Check sheet for the modelled part. Datum: model origin and axes. Units: mm. Face numbers are marked on the shaded views. Give positions to 0.01 mm unless a question says otherwise; leave off trailing zeros. Loops run counter-clockwise (first coordinate to the right, second up) from the corner with the lowest first, then second, coordinate; pieces in that order, holes last. Notation, with made-up numbers: (35, -5.75) - (73, -5.75) arc R34 ccw to (73, 27.25) - close; hole circle Ø7 at (-20, -3.75). An arc over 180 degrees is marked (long way). Use one line per item in the form item = value.
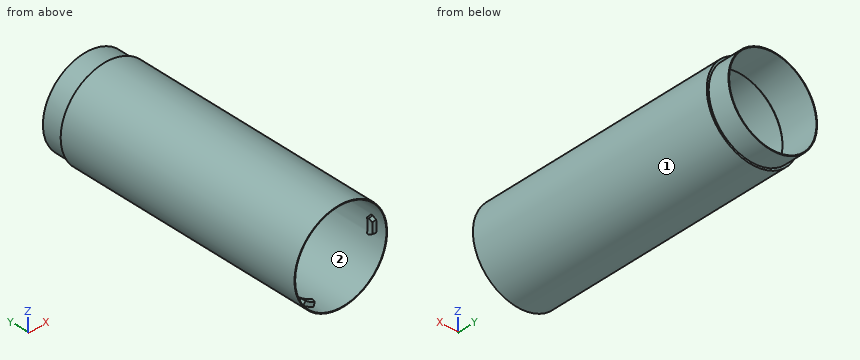
Autodesk Inventor part; units mm, degrees
ref_plane "Work Plane2" through (35, 0, 0) normal (1, 0, 0) x (0, 1, 0)
ref_plane "Work Plane4" through (34, 0, 0) normal (1, 0, 0) x (0, 1, 0)
ref_plane "Work Plane5" through (0, 8, 0) normal (0, -1, 0) x (1, 0, 0)
sketch "Sketch1" plane through (0, 0, 0) normal (0, 1, 0) x (-1, 0, 0)
  circle A0 centre (0, 0) radius 35
  circle A1 centre (0, 0) radius 34.5
  dimension "d0" = 70
  dimension "d1" = 69
extrude "Extrusion1" add sketch "Sketch1" along normal blind 189.5
ref_plane "Work Plane2" through (35, 0, 0) normal (1, 0, 0) x (0, 1, 0)
sketch "Sketch5" plane through (0, 189.5, 0) normal (0, 1, 0) x (1, 0, 0)
  circle A0 centre (0, 0) radius 33.5
  circle A1 centre (0, 0) radius 33
  dimension "d44" = 67
  dimension "d45" = 66
extrude "Extrusion3" add sketch "Sketch5" along normal blind 16
sketch "Sketch6" plane through (0, 189.5, 0) normal (0, -1, 0) x (1, 0, 0)
  circle A0 centre (0, 0) radius 33
  circle A1 centre (0, 0) radius 34.5
  circle A2 centre (0, 0) radius 34.5
  dimension "d112" = 66
  dimension "d113" = 69
extrude "Extrusion4" add sketch "Sketch6" along normal blind 12.5
ref_plane "Work Plane4" through (34, 0, 0) normal (1, 0, 0) x (0, 1, 0)
ref_plane "Work Plane5" through (0, 8, 0) normal (0, -1, 0) x (1, 0, 0)
sketch "Sketch11" plane through (0, 8, 0) normal (0, -1, 0) x (1, 0, 0)
  line L0 (0, 0) -> (37.8059, -6.6662) construction
  line L1 (37.8059, 6.6662) -> (0, 0) construction
  line L2 (0, 0) -> (37.8692, 0) construction
  arc A0 (33.9759, -5.9909) -> (33.9759, 5.9909) centre (0, 0) ccw
  arc A1 (31.0214, -5.4699) -> (31.0214, 5.4699) centre (0, 0) ccw
  line L3 (31.0214, 5.4699) -> (33.9759, 5.9909)
  line L4 (31.0214, -5.4699) -> (33.9759, -5.9909)
  dimension "d94" = 10
  dimension "d95" = 10
  dimension "d96" = 34.5
  dimension "d97" = 31.5
extrude "Extrusion5" add sketch "Sketch11" against normal blind 4
chamfer "Chamfer1" distance 1.5 angle 60 2 edges at (32.4987, 8, -5.7304) (32.4987, 8, 5.7304) measured on face at (33.4433, 8, -0.6105)
pattern_circular "Circular Pattern4" count 3 over 360 about axis through (0, 0, 0) along (0, 1, 0) of "Extrusion5", "Chamfer1"
ref_plane "Work Plane6" through (0, 25, 0) normal (0, -1, 0) x (1, 0, 0)
chamfer "Chamfer2" distance 1 angle 45 1 edges at (-33, 177, 0)
properties part number "Engine skin" material "Plastic, Opaque White"
Item 1: Section check A-A on x = 0. Record the boundary of the cut face in (y, z).
Answer block:
outline = (0, -35) - (189.5, -35) - (189.5, -33.5) - (205.5, -33.5) - (205.5, -33) - (178, -33) - (177, -34) - (177, -34.5) - (0, -34.5) - close; (0, 34.5) - (177, 34.5) - (177, 34) - (178, 33) - (205.5, 33) - (205.5, 33.5) - (189.5, 33.5) - (189.5, 35) - (0, 35) - close
Item 2: Thickness scan on L1, parallel to Z at x = 0, y = 195.25; L2, parallel to Z at x = -0.5, y = 19.5; L3, parallel to X at y = 49, z = -6. Record the ranges inside material, lowest first.
Answer block:
L1 = -33.5 to -33, 33 to 33.5
L2 = -35 to -34.5, 34.5 to 35
L3 = -34.48 to -33.97, 33.97 to 34.48
Item 3: Section check B-B on z = 0. Record the boundary of the cut face in (x, y), then the cut area to 3 significant figures.
Answer block:
outline = (-35, 0) - (-34.5, 0) - (-34.5, 177) - (-34, 177) - (-33, 178) - (-33, 205.5) - (-33.5, 205.5) - (-33.5, 189.5) - (-35, 189.5) - close; (31.5, 8) - (34.5, 8) - (34.5, 0) - (35, 0) - (35, 189.5) - (33.5, 189.5) - (33.5, 205.5) - (33, 205.5) - (33, 178) - (34, 177) - (34.5, 177) - (34.5, 12) - (31.5, 12) - close
area = 254 mm2
Item 4: Section check C-C on y = 30.5. Record the boundary of the cut face in (x, z).
Answer block:
outline = circle Ø70 at (0, 0); hole circle Ø69 at (0, 0)
Item 5: Gauge pin test, flat ends, axial feed: P1, Ø1, axis at y = 54.5, z = -8, coming from the +X side; P2, Ø8, axis at x = -6, y = 48.5, coming from the -Z side; P3, Ø1, axis at y = 20.5, z = -3.5, coming from the -X side. Record the tip position at first contact, or that the pin passes through.
Answer block:
P1 = 34.19
P2 = -34.94
P3 = -34.87
Item 6: Mould release check, pull along Y, two halves, no side actions. Record for the marked faces 1 and 2: released by +Y, released by -Y, zero draft, split by the parting line, or undercut.
Answer block:
face_1 = zero draft
face_2 = undercut
